Verification items for the finished model (mm, model axes). A direction names the side the tool comes from. Round coordinates to 2 decimals unless told otherwise and drop trailing zeros. Order: outer loops, then holes, each group sorted by start corner. A loop starts at its lowest first (then second) coordinate and runs counter-clockwise, first axis right, second up. Notation, with made-up numbers: (7.25, 70.5) -> (49.25, 70.5) arc R29 cw to (49.25, 94.5) -> close; hole circle Ø3 at (28, -11). An arc over 180 degrees is marked (long way). Return JSON: item names as keys, results as strings. Group by question number.
Item 1: Depth check by flat-ended pin: pin 1 Ø1.5 at (x, y) = (-1, -28.5) entering from +Z; pin 2 Ø10 at (x, z) = (-16.5, 15) entering from -Y; pin 3 Ø1.5 at (y, z) = (-26, 16) entering from -X. Enter the tip coordinate at first touch or a pass-through.
Item 2: Sectioned sample at C-C on y = 0. Record the cut outline in (x, z), plus the area to 3 significant figures.
Item 3: Sectioned sample at A-A on z = 16.25. Record the cut outline in (x, y), plus the area to 3 significant figures.
Item 4: Sectioned sample at B-B on z = 4.75. Give the number of separate pieces and of enclosed holes in the cut face, plus the area to 3 significant figures.
Item 5: Draft check along Y on faces 4 (the flat face through (18.29, 29.16, 13.92)), 5 (the flat face through (9, 28, 16)), 6 (the cylindrical face through (21.59, 12.61, 13.92)), 7 (the cylindrical face through (2.05, -13.54, 5.07)). Enter one of: pulls with the +Y half, pulls with the -Y half, needs draft (parallel to the pull), parting line crosses it, or undercut.
Item 6: Access from +Z, -Z, +X, -X, +Y, -Y to the whole of each face (thin tool, end or side, straight path). Record for faces 1 (the flat face through (-28.26, -9.39, 12.77)), 2 (the flat face through (-19.98, -21.93, 15.98)), 3 (the flat face through (6, 29, 13)).
Item 7: Scan lines: probe 1 along Y at (x, z) = (0, 4); probe 2 along X at (y, z) = (7, 6.5); probe 3 along Y at (x, z) = (27.5, 3.25). Record each from-to range of solid material in increasing order. Write a range as from..to.
```python
from build123d import *

# Parameters (mm, degrees)
SKETCH1_R               = 40
BOSS_EXTRUDE1_DEPTH     = 20
CUT_EXTRUDE1_START      = -12
CUT_EXTRUDE1_DEPTH      = 12
CIRPATTERN1_COUNT       = 3
CIRPATTERN2_COUNT       = 3
CIRPATTERN3_COUNT       = 3
M6_TAPPED_HOLE2_D       = 5
CHAMFER1_SIZE           = 1
CUT_EXTRUDE2_REACH      = 62
CUT_EXTRUDE2_END_RADIUS = 40
CIRPATTERN4_COUNT       = 3
CHAMFER2_SIZE           = 1


with BuildPart() as part:
    # Sketch1 → Boss-Extrude1 (new body)
    with BuildSketch(Plane.XY):
        Circle(SKETCH1_R)
    extrude(amount=BOSS_EXTRUDE1_DEPTH)

    # Sketch2 → Cut-Extrude1 (cut)
    with BuildSketch(Plane.XY.offset(20).offset(CUT_EXTRUDE1_START)):
        with BuildLine():
            Line((-39.331070493, -7.284702732), (-29.329853145, 10.037913852))
            ThreePointArc((-29.329853145, 10.037913852), (-21.650635095, 12.5), (-23.358014969, 20.381440987))
            Line((-23.358014969, 20.381440987), (-13.356797621, 37.704057571))
            ThreePointArc((-13.356797621, 37.704057571), (-34.641016151, 20), (-39.331070493, -7.284702732))
        make_face()
    cut_extrude1 = extrude(amount=CUT_EXTRUDE1_DEPTH, mode=Mode.SUBTRACT)

    # CirPattern1: Cut-Extrude1 ×3 about axis
    cirpattern1_axis = Axis((0, 0, 0), (0, 0, 1))
    for i in range(1, CIRPATTERN1_COUNT):
        add(cut_extrude1.rotate(cirpattern1_axis, i * 360 / CIRPATTERN1_COUNT), mode=Mode.SUBTRACT)

    # Sketch3 → Cut-Revolve1 (revolve, cut)
    with BuildSketch(Plane(origin=(0, 0, 0), x_dir=(0, 0, -1), z_dir=(1, 0, 0)), mode=Mode.PRIVATE) as cut_revolve1_sk:
        Polygon((-20, 0), (-20, 20), (-10, 20), (-10, 9), (0, 9), (0, 0), align=None)
    revolve(cut_revolve1_sk.sketch.rotate(Axis((0, 0, 0), (0, 0, 1)), 90), axis=Axis((0, 0, 0), (0, 0, 1)), mode=Mode.SUBTRACT)

    # Sketch7 → M5 Tapped Hole1 (revolve, cut)
    with BuildSketch(Plane(origin=(0, -14, 10), x_dir=(0, -1, 0), z_dir=(1, 0, 0))):
        Polygon((0, 0), (0, 14), (2.1, 12.7381927), (2.1, 0), align=None)
    m5_tapped_hole1 = revolve(axis=Axis((0, -14, 16.35), (0, 0, -1)), mode=Mode.SUBTRACT)

    # CirPattern2: M5 Tapped Hole1 ×3 about axis
    cirpattern2_axis = Axis((0, 0, 0), (0, 0, 1))
    for i in range(1, CIRPATTERN2_COUNT):
        add(m5_tapped_hole1.rotate(cirpattern2_axis, i * 360 / CIRPATTERN2_COUNT), mode=Mode.SUBTRACT)

    # Sketch9 → M8 Tapped Hole1 (revolve, cut)
    with BuildSketch(Plane(origin=(-26.846787517, 15.5, 8), x_dir=(0, -1, 0), z_dir=(1, 0, 0))):
        Polygon((0, 0), (0, 22.25), (3.4, 20.207073895), (3.4, 0), align=None)
    m8_tapped_hole1 = revolve(axis=Axis((-26.846787517, 15.5, 14.35), (0, 0, -1)), mode=Mode.SUBTRACT)

    # CirPattern3: M8 Tapped Hole1 ×3 about axis
    cirpattern3_axis = Axis((0, 0, 0), (0, 0, 1))
    for i in range(1, CIRPATTERN3_COUNT):
        add(m8_tapped_hole1.rotate(cirpattern3_axis, i * 360 / CIRPATTERN3_COUNT), mode=Mode.SUBTRACT)

    # M6 Tapped Hole2 (through all)
    with Locations(Plane.XY.offset(20)):
        with Locations((25.980762114, -15)):
            Hole(M6_TAPPED_HOLE2_D / 2)

    # Chamfer1
    chamfer1_edges = [part.edges().sort_by_distance(p)[0] for p in [
        (20, 0, 20),
        (20, 0, 10),
    ]]
    chamfer(chamfer1_edges, length=CHAMFER1_SIZE)

    # Cut-Extrude2: up to this cylinder (the profile starts inside it)
    cut_extrude2_end = Plane(origin=(0, 0, 15.805147), z_dir=(0, 0, -1)) * Cylinder(CUT_EXTRUDE2_END_RADIUS, 205, mode=Mode.PRIVATE)
    # Sketch12 → Cut-Extrude2 (cut, up to the surface)
    with BuildSketch(Plane(origin=(0, 0, 0), x_dir=(1, 0, 0), z_dir=(0, 1, 0)), mode=Mode.PRIVATE) as cut_extrude2_sk1:
        Polygon((8, -20), (8, -17.5), (9, -17.5), (9, -14.5), (6, -14.5), (6, -11), (-6, -11), (-6, -14.5), (-9, -14.5), (-9, -17.5), (-8, -17.5), (-8, -20), align=None)
    cut_extrude2_tool1 = extrude(cut_extrude2_sk1.sketch, amount=CUT_EXTRUDE2_REACH, mode=Mode.PRIVATE) & cut_extrude2_end
    cut_extrude2 = cut_extrude2_tool1.solids().sort_by_distance((0, 0, 15.805147))[0]
    add(cut_extrude2, mode=Mode.SUBTRACT)

    # CirPattern4: Cut-Extrude2 ×3 about axis
    cirpattern4_axis = Axis((0, 0, 0), (0, 0, 1))
    for i in range(1, CIRPATTERN4_COUNT):
        add(cut_extrude2.rotate(cirpattern4_axis, i * 360 / CIRPATTERN4_COUNT), mode=Mode.SUBTRACT)

    # Chamfer2
    chamfer2_edges = [part.edges().sort_by_distance(p)[0] for p in [
        (9, 0, 10),
    ]]
    chamfer(chamfer2_edges, length=CHAMFER2_SIZE)


solid = part.part
```
Recorded:
{
 "1": {"pin 1": "z = 8", "pin 2": "y = -30.42", "pin 3": "x = -28.33"},
 "2": {"outline": "(-40, 0) -> (-9, 0) -> (-9, 9) -> (-10, 10) -> (-19, 10) -> (-20, 11) -> (-20, 19) -> (-21, 20) -> (-35.13, 20) -> (-35.13, 8) -> (-40, 8) -> close; (9, 0) -> (40, 0) -> (40, 8) -> (35.13, 8) -> (35.13, 20) -> (21, 20) -> (20, 19) -> (20, 11) -> (19, 10) -> (10, 10) -> (9, 9) -> close", "area": "902 mm²"},
 "3": {"outline": "(-39.33, -7.28) arc R40 ccw to (-38.25, -11.69) -> (-19.97, -1.14) arc R20 cw to (-9, 17.86) -> (-9, 38.97) arc R40 ccw to (-13.36, 37.7) -> (-23.36, 20.38) arc R6 cw to (-29.33, 10.04) -> close; (-29.25, -27.28) arc R40 ccw to (-25.97, -30.42) -> (-5.97, -30.42) arc R6 cw to (5.97, -30.42) -> (25.97, -30.42) arc R40 ccw to (29.25, -27.28) -> (10.97, -16.72) arc R20 cw to (-10.97, -16.72) -> close; (9, 17.86) arc R20 cw to (19.97, -1.14) -> (38.25, -11.69) arc R40 ccw to (39.33, -7.28) -> (29.33, 10.04) arc R6 cw to (23.36, 20.38) -> (13.36, 37.7) arc R40 ccw to (9, 38.97) -> close", "area": "1,500 mm²"},
 "4": {"separate pieces": "1", "enclosed holes": "8", "area": "4,600 mm²"},
 "5": {"face 4": "pulls with the +Y half", "face 5": "needs draft", "face 6": "undercut", "face 7": "undercut"},
 "6": {"face 1": "+Z", "face 2": "-X", "face 3": "+Z, +Y"},
 "7": {"probe 1": "-40..-34.4, -27.6..-16.1, -11.9..-9, 9..40", "probe 2": "-39.38..-14.22, -10.02..-5.66, 5.66..10.02, 14.22..39.38", "probe 3": "-29.05..-16.99, -13.01..12.16, 18.84..29.05"}
}
